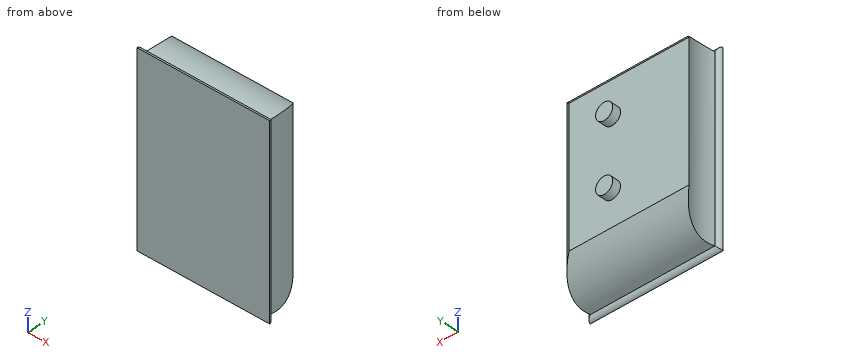
```python
from build123d import *

# Parameters (mm, degrees)
SKETCH1_W               = 228.6
SKETCH1_H               = 101.6
BOSS_EXTRUDE1_DEPTH     = 38.1
SKETCH2_W               = 266.7
SKETCH2_H               = 139.7
BOSS_EXTRUDE2_DEPTH     = 38.1
CUT_EXTRUDE1_DEPTH      = 70.85
CUT_EXTRUDE1_DEPTH_BACK = 70.85
CUT_EXTRUDE2_DEPTH      = 134.35
CUT_EXTRUDE2_DEPTH_BACK = 134.35
BOSS_EXTRUDE3_DEPTH     = 117.475
CUT_EXTRUDE3_DEPTH      = 70.85
CUT_EXTRUDE3_DEPTH_BACK = 70.85
BOSS_EXTRUDE6_DEPTH     = 50.8
CUT_EXTRUDE4_DEPTH      = 134.35
CUT_EXTRUDE4_DEPTH_BACK = 134.35
BOSS_EXTRUDE7_DEPTH     = 11.43
SKETCH12_W              = 101.6
SKETCH12_H              = 44.45
CUT_EXTRUDE5_DEPTH      = 57.15
SKETCH13_W              = 25.4
SKETCH13_H              = 15.875
CUT_EXTRUDE6_DEPTH      = 8.89
SKETCH14_W              = 234.95
SKETCH14_H              = 73.385904338
CUT_EXTRUDE7_DEPTH      = 70.85
CUT_EXTRUDE7_DEPTH_BACK = 70.85
SKETCH15_R              = 6.35
BOSS_EXTRUDE8_DEPTH     = 6.35
SKETCH16_W              = 114.519931472
SKETCH16_H              = 54.078527613
CUT_EXTRUDE8_DEPTH      = 70.85
CUT_EXTRUDE8_DEPTH_BACK = 70.85


with BuildPart() as part:
    # Sketch1 → Boss-Extrude1 (new body)
    with BuildSketch(Plane(origin=(0, 0, 0), x_dir=(1, 0, 0), z_dir=(0, 1, 0))):
        Rectangle(SKETCH1_W, SKETCH1_H)
    extrude(amount=BOSS_EXTRUDE1_DEPTH)

    # Sketch2 → Boss-Extrude2 (add)
    with BuildSketch(Plane.XZ):
        Rectangle(SKETCH2_W, SKETCH2_H)
    extrude(amount=BOSS_EXTRUDE2_DEPTH)

    # Sketch4 → Cut-Extrude1 (cut, two sides)
    with BuildSketch(Plane.XY) as cut_extrude1_sk:
        with BuildLine():
            Line((25.4, 0), (-25.4, 0))
            ThreePointArc((-25.4, 0), (-36.780856653, -15.633097581), (-38.1, -34.925))
            ThreePointArc((-38.1, -34.925), (-35.85493597, -35.85493597), (-34.925, -38.1))
            Line((-34.925, -38.1), (34.925, -38.1))
            ThreePointArc((34.925, -38.1), (35.85493597, -35.85493597), (38.1, -34.925))
            ThreePointArc((38.1, -34.925), (36.780856653, -15.633097581), (25.4, 0))
        make_face()
        with BuildLine():
            Line((114.3, 0), (138.625991559, 8.381745969))
            Line((138.625991559, 8.381745969), (149.850712343, -24.19529276))
            Line((149.850712343, -24.19529276), (133.35, -38.1))
            ThreePointArc((133.35, -38.1), (132.42006403, -35.85493597), (130.175, -34.925))
            ThreePointArc((130.175, -34.925), (127.462245798, -15.087615547), (114.3, 0))
        make_face()
        with BuildLine():
            Line((-149.850712343, -24.19529276), (-133.35, -38.1))
            ThreePointArc((-133.35, -38.1), (-132.42006403, -35.85493597), (-130.175, -34.925))
            ThreePointArc((-130.175, -34.925), (-127.462245798, -15.087615547), (-114.3, 0))
            Line((-114.3, 0), (-138.625991559, 8.381745969))
            Line((-138.625991559, 8.381745969), (-149.850712343, -24.19529276))
        make_face()
    extrude(amount=CUT_EXTRUDE1_DEPTH, mode=Mode.SUBTRACT)
    extrude(cut_extrude1_sk.sketch, amount=-CUT_EXTRUDE1_DEPTH_BACK, mode=Mode.SUBTRACT)

    # Sketch5 → Cut-Extrude2 (cut, two sides)
    with BuildSketch(Plane(origin=(0, 0, 0), x_dir=(0, 0, -1), z_dir=(1, 0, 0))) as cut_extrude2_sk:
        with BuildLine():
            Line((-69.85, -38.1), (-80.267672211, -6.179959038))
            Line((-80.267672211, -6.179959038), (-69.85, 0.848763613))
            Line((-69.85, 0.848763613), (-50.8, 0))
            ThreePointArc((-50.8, 0), (-63.962245798, -15.087615547), (-66.675, -34.925))
            ThreePointArc((-66.675, -34.925), (-68.92006403, -35.85493597), (-69.85, -38.1))
        make_face()
        with BuildLine():
            Line((69.85, 0.848763613), (50.8, 0))
            ThreePointArc((50.8, 0), (63.962245798, -15.087615547), (66.675, -34.925))
            ThreePointArc((66.675, -34.925), (68.92006403, -35.85493597), (69.85, -38.1))
            Line((69.85, -38.1), (80.267672211, -6.179959038))
            Line((80.267672211, -6.179959038), (69.85, 0.848763613))
        make_face()
    extrude(amount=CUT_EXTRUDE2_DEPTH, mode=Mode.SUBTRACT)
    extrude(cut_extrude2_sk.sketch, amount=-CUT_EXTRUDE2_DEPTH_BACK, mode=Mode.SUBTRACT)

    # Sketch7 → Boss-Extrude3 (add, symmetric)
    with BuildSketch(Plane(origin=(0, 0, 0), x_dir=(0, 0, -1), z_dir=(1, 0, 0))):
        with BuildLine():
            Line((-50.8, 38.1), (50.8, 38.1))
            ThreePointArc((50.8, 38.1), (53.975, 34.925), (50.8, 31.75))
            ThreePointArc((50.8, 31.75), (52.363441445, 19.05), (50.8, 6.35))
            ThreePointArc((50.8, 6.35), (53.975, 3.175), (50.8, 0))
            Line((50.8, 0), (-50.8, 0))
            ThreePointArc((-50.8, 0), (-53.975, 3.175), (-50.8, 6.35))
            ThreePointArc((-50.8, 6.35), (-52.363441445, 19.05), (-50.8, 31.75))
            ThreePointArc((-50.8, 31.75), (-53.975, 34.925), (-50.8, 38.1))
        make_face()
    extrude(amount=BOSS_EXTRUDE3_DEPTH, both=True)

    # Sketch8 → Cut-Extrude3 (cut, two sides)
    with BuildSketch(Plane.XY) as cut_extrude3_sk:
        with BuildLine():
            Line((-114.3, 38.1), (-123.468271352, 41.287608438))
            Line((-123.468271352, 41.287608438), (-120.491237125, -2.317187004))
            Line((-120.491237125, -2.317187004), (-114.3, 0))
            ThreePointArc((-114.3, 0), (-117.475, 3.175), (-114.3, 6.35))
            ThreePointArc((-114.3, 6.35), (-116.592108499, 19.05), (-114.3, 31.75))
            ThreePointArc((-114.3, 31.75), (-117.475, 34.925), (-114.3, 38.1))
        make_face()
        with BuildLine():
            Line((120.491237125, -2.317187004), (114.3, 0))
            ThreePointArc((114.3, 0), (117.475, 3.175), (114.3, 6.35))
            ThreePointArc((114.3, 6.35), (116.592108499, 19.05), (114.3, 31.75))
            ThreePointArc((114.3, 31.75), (117.475, 34.925), (114.3, 38.1))
            Line((114.3, 38.1), (123.468271352, 41.287608438))
            Line((123.468271352, 41.287608438), (120.491237125, -2.317187004))
        make_face()
    extrude(amount=CUT_EXTRUDE3_DEPTH, mode=Mode.SUBTRACT)
    extrude(cut_extrude3_sk.sketch, amount=-CUT_EXTRUDE3_DEPTH_BACK, mode=Mode.SUBTRACT)

    # Sketch9 → Boss-Extrude6 (add, symmetric)
    with BuildSketch(Plane.XY):
        with BuildLine():
            Line((-114.3, 38.1), (114.3, 38.1))
            ThreePointArc((114.3, 38.1), (92.707665567, 45.121477655), (79.375, 63.5))
            ThreePointArc((79.375, 63.5), (0, 41.272917837), (-79.375, 63.5))
            ThreePointArc((-79.375, 63.5), (-92.707665567, 45.121477655), (-114.3, 38.1))
        make_face()
    extrude(amount=BOSS_EXTRUDE6_DEPTH, both=True)

    # Sketch10 → Cut-Extrude4 (cut, two sides)
    with BuildSketch(Plane(origin=(0, 0, 0), x_dir=(0, 0, -1), z_dir=(1, 0, 0))) as cut_extrude4_sk:
        with BuildLine():
            Line((25.4, 63.5), (50.8, 63.5))
            Line((50.8, 63.5), (50.8, 38.1))
            ThreePointArc((50.8, 38.1), (35.780017166, 48.480017166), (25.4, 63.5))
        make_face()
        with BuildLine():
            Line((-50.8, 63.5), (-50.8, 38.1))
            ThreePointArc((-50.8, 38.1), (-35.780017166, 48.480017166), (-25.4, 63.5))
            Line((-25.4, 63.5), (-50.8, 63.5))
        make_face()
    extrude(amount=CUT_EXTRUDE4_DEPTH, mode=Mode.SUBTRACT)
    extrude(cut_extrude4_sk.sketch, amount=-CUT_EXTRUDE4_DEPTH_BACK, mode=Mode.SUBTRACT)

    # Sketch11 → Boss-Extrude7 (add)
    with BuildSketch(Plane.XY.offset(9.525)):
        with BuildLine():
            Line((-79.375, 63.5), (-79.375, 68.58))
            ThreePointArc((-79.375, 68.58), (0, 45.590721784), (79.375, 68.58))
            Line((79.375, 68.58), (79.375, 63.5))
            ThreePointArc((79.375, 63.5), (0, 23.789706403), (-79.375, 63.5))
        make_face()
    extrude(amount=BOSS_EXTRUDE7_DEPTH)

    # Sketch12 → Cut-Extrude5 (cut)
    with BuildSketch(Plane(origin=(0, 63.5, 0), x_dir=(-1, 0, 0), z_dir=(0, -1, 0))):
        Rectangle(SKETCH12_W, SKETCH12_H)
    extrude(amount=CUT_EXTRUDE5_DEPTH, mode=Mode.SUBTRACT)

    # Sketch13 → Cut-Extrude6 (cut)
    with BuildSketch(Plane.XY.offset(-22.225)):
        with Locations((-6.35, 26.9875)):
            Rectangle(SKETCH13_W, SKETCH13_H)
    extrude(amount=-CUT_EXTRUDE6_DEPTH, mode=Mode.SUBTRACT)

    # Sketch14 → Cut-Extrude7 (cut, two sides)
    with BuildSketch(Plane.XY) as cut_extrude7_sk:
        with Locations((0, 36.692952169)):
            Rectangle(SKETCH14_W, SKETCH14_H)
    extrude(amount=CUT_EXTRUDE7_DEPTH, mode=Mode.SUBTRACT)
    extrude(cut_extrude7_sk.sketch, amount=-CUT_EXTRUDE7_DEPTH_BACK, mode=Mode.SUBTRACT)

    # Sketch15 → Boss-Extrude8 (add)
    with BuildSketch(Plane(origin=(0, 0, 0), x_dir=(1, 0, 0), z_dir=(0, 1, 0))):
        with Locations(Location((-82.55, 25.4, 0), (0, 0, 90))):  # turned: the seam where the file's is
            Circle(SKETCH15_R)
        with Locations(Location((-82.55, -25.4, 0), (0, 0, 90))):  # turned: the seam where the file's is
            Circle(SKETCH15_R)
        with Locations(Location((82.55, -25.4, 0), (0, 0, 90))):  # turned: the seam where the file's is
            Circle(SKETCH15_R)
        with Locations(Location((82.55, 25.4, 0), (0, 0, 90))):  # turned: the seam where the file's is
            Circle(SKETCH15_R)
    extrude(amount=BOSS_EXTRUDE8_DEPTH)

    # Sketch16 → Cut-Extrude8 (cut, two sides)
    with BuildSketch(Plane.XY) as cut_extrude8_sk:
        with Locations((-80.803403424, -19.002671916)):
            Rectangle(SKETCH16_W, SKETCH16_H)
    extrude(amount=CUT_EXTRUDE8_DEPTH, mode=Mode.SUBTRACT)
    extrude(cut_extrude8_sk.sketch, amount=-CUT_EXTRUDE8_DEPTH_BACK, mode=Mode.SUBTRACT)


solid = part.part
```
Work out the finished part from the listing and answer in its coordinate system (mm). Round coordinates to 2 decimals unless told otherwise and drop trailing zeros. Write each loop counter-clockwise with the first axis right and the second up, starting at its lowest first coordinate (ties: lowest second). Pieces come first, ordered by that corner, then holes. Notation, with made-up numbers: (60.5, 58) - (114.5, 58) arc R26 ccw to (114.5, 76) - close; hole circle Ø9 at (77.5, 1). An arc over 180 degrees is marked (long way). Return JSON: item names as keys, results as strings. Group by question number.
Q1. The part is cut by section D-D on z = -48. Write down the section's boundary in (x, y) (3 decimals), then the cut area to 3 significant figures.
Q2. Each of these flat-tipped pins is pushed along its axis until it touches: pin 1 Ø6 at (y, z) = (-6.5, 9) entering from -X; pin 2 Ø8 at (y, z) = (-27, -25.5) entering from -X; pin 3 Ø1.5 at (x, y) = (46.5, -19) entering from +Z. Where does it stop, or does it pass through?
Q3. The part is cut by section B-B on z = 25. Write down the section's boundary in (x, y) (3 decimals), then the cut area to 3 significant figures.
Q4. The part is cut by section C-C on y = -2. Write down the section's boundary in (x, z), then the cut area to 3 significant figures.
Q5. The part is cut by section A-A on x = 82.55. Write down the section's boundary in (y, z) (3 decimals), then the cut area to 3 significant figures.
Q6. Find the intervals of material crossed by L1, parallel to Y at x = 97, z = 6.5; L2, parallel to Z at x = 99.5, y = -29.5; L3, parallel to Z at x = 46, y = -16.5, in increasing order.
Solved:
{
 "1": {"outline": "(25.4, 0) arc R34.925 cw to (38.1, -34.925) arc R3.175 ccw to (34.925, -38.1) - (133.35, -38.1) arc R3.175 ccw to (130.175, -34.925) arc R34.925 ccw to (114.3, 0) - close", "area": "3,480 mm²"},
 "2": {"pin 1": "x = 29.27", "pin 2": "x = 38.58", "pin 3": "z = 65.69"},
 "3": {"outline": "(25.4, 0) arc R34.925 cw to (38.1, -34.925) arc R3.175 ccw to (34.925, -38.1) - (133.35, -38.1) arc R3.175 ccw to (130.175, -34.925) arc R34.925 ccw to (114.3, 0) - (88.887, 0) - (88.887, 6.35) - (76.213, 6.35) - (76.213, 0) - close", "area": "3,560 mm²"},
 "4": {"outline": "(27.75, -53.65) - (117.15, -53.65) - (117.15, 53.65) - (27.75, 53.65) - close", "area": "9,590 mm²"},
 "5": {"outline": "(-38.1, -69.85) arc R3.175 ccw to (-34.925, -66.675) arc R34.925 ccw to (0, -50.8) - (0, -31.75) - (6.35, -31.75) - (6.35, -19.05) - (0, -19.05) - (0, 19.05) - (6.35, 19.05) - (6.35, 31.75) - (0, 31.75) - (0, 50.8) arc R34.925 ccw to (-34.925, 66.675) arc R3.175 ccw to (-38.1, 69.85) - close", "area": "5,000 mm²"},
 "6": {"L1": "-38.1 to 0", "L2": "-67.09 to 67.09", "L3": "-64.57 to 64.57"}
}
